Read the model definition and answer for the solid it produces. Units are mm, in the model's axes. A direction names the side the tool comes from. Round coordinates to 2 decimals unless told otherwise and drop trailing zeros. Write each loop counter-clockwise with the first axis right and the second up, starting at its lowest first coordinate (ties: lowest second). Pieces come first, ordered by that corner, then holes. Notation, with made-up numbers: (14.5, 22.5) -> (55.5, 22.5) arc R7 ccw to (55.5, 30.5) -> close; hole circle Ø5 at (-35, -32). An arc over 180 degrees is marked (long way). Return JSON: item names as keys, results as strings. Group by question number.
(1) Given pin 1 (1 mm diameter, centred on y = 4.5, z = 21.5, fed in from -X), flat-ended and moving along its own axis, determine where the tip first touches the part or whether it passes through.
(2) Straight lines are drawn through the part: line 1 (X direction, y = 0.25, z = 16.5); line 2 (Z direction, x = 4.25, y = 4.75); line 3 (Y direction, x = 0, z = -11.5). For each, find the intervals that lie inside material, in ascending order.
(3) The mould has two halves that part along Y. Classify faces 1 (the flat face through (0, 6.35, 1)), 2 (the cylindrical face through (1.926, 0.607, 1.451)), 3 (the flat face through (3, -6, 67.443)): released by +Y, released by -Y, zero draft, split by the parting line, or undercut.
(4) A cutting plane is placed at A-A on z = -51.5. Give the vertices of the cut face in (x, y) (3 decimals), then the cut area to 3 significant figures.
(5) For faces 4 (the flat face through (-1, 2, 67.443)), 5 (the flat face through (-3, 6, 67.443)), 6 (the flat face through (-3, -6, 67.443)), determine the directions among +Z, -Z, +X, -X, +Y, -Y from which every point of the face is accessible in a straight line to the end or side of a thin tool.
```python
from build123d import *

# Parameters (mm, degrees)
BOSS_EXTRUDE1_DEPTH              = 67.44335
SKETCH4_R                        = 6.35
SKETCH4_R_2                      = 2.4892
BOSS_EXTRUDE2_DEPTH              = 7.9375
F_10_32_TAPPED_HOLE1_D           = 4.0386
F_10_32_TAPPED_HOLE1_CSINK_D     = 6.096
F_10_32_TAPPED_HOLE1_CSINK_ANGLE = 90


with BuildPart() as part:
    # Sketch1 → Boss-Extrude1 (new, symmetric)
    with BuildSketch(Plane.XY):
        with BuildLine():
            ThreePointArc((4.181770846, 5.456960429), (3.437499983, 5.953924622), (2.634980936, 6.35))
            Line((2.634980936, 6.35), (-2.634980936, 6.35))
            ThreePointArc((-2.634980936, 6.35), (-3.437499983, 5.953924622), (-4.181770846, 5.456960429))
            Line((-4.181770846, 5.456960429), (-6.816751782, 0.893039571))
            ThreePointArc((-6.816751782, 0.893039571), (-6.874999966, 0), (-6.816751782, -0.893039571))
            Line((-6.816751782, -0.893039571), (-4.181770846, -5.456960429))
            ThreePointArc((-4.181770846, -5.456960429), (-3.437499983, -5.953924622), (-2.634980936, -6.35))
            Line((-2.634980936, -6.35), (2.634980936, -6.35))
            ThreePointArc((2.634980936, -6.35), (3.437499983, -5.953924622), (4.181770846, -5.456960429))
            Line((4.181770846, -5.456960429), (6.816751782, -0.893039571))
            ThreePointArc((6.816751782, -0.893039571), (6.860422465, -0.447468582), (6.874999966, 0))
            ThreePointArc((6.874999966, 0), (6.860422465, 0.447468582), (6.816751782, 0.893039571))
            Line((6.816751782, 0.893039571), (4.181770846, 5.456960429))
        make_face()
    extrude(amount=BOSS_EXTRUDE1_DEPTH, both=True)

    # Sketch4 → Boss-Extrude2 (add)
    with BuildSketch(Plane.XY.offset(67.44335)):
        with Locations(Location((0, 0, 0), (0, 0, 150))):
            Circle(SKETCH4_R)
        Circle(SKETCH4_R_2, mode=Mode.SUBTRACT)
    extrude(amount=BOSS_EXTRUDE2_DEPTH)

    # #10-32 Tapped Hole1 (through all)
    with Locations(Plane(origin=(0, 0, -67.44335), x_dir=(-1, 0, 0), z_dir=(0, 0, -1))):
        with Locations((0, 0)):
            CounterSinkHole(F_10_32_TAPPED_HOLE1_D / 2, F_10_32_TAPPED_HOLE1_CSINK_D / 2, counter_sink_angle=F_10_32_TAPPED_HOLE1_CSINK_ANGLE)


solid = part.part
```
Checks:
{
 "1": {"pin 1": "stops at x = -5.02"},
 "2": {"line 1": "x = -6.87 to -2, 2 to 6.87", "line 2": "z = -67.44 to 67.44", "line 3": "y = -6.35 to -2.02, 2.02 to 6.35"},
 "3": {"face 1": "released by +Y", "face 2": "undercut", "face 3": "zero draft"},
 "4": {"outline": "(-6.817, -0.893) -> (-4.182, -5.457) arc R6.875 ccw to (-2.635, -6.35) -> (2.635, -6.35) arc R6.875 ccw to (4.182, -5.457) -> (6.817, -0.893) arc R6.875 ccw to (6.817, 0.893) -> (4.182, 5.457) arc R6.875 ccw to (2.635, 6.35) -> (-2.635, 6.35) arc R6.875 ccw to (-4.182, 5.457) -> (-6.817, 0.893) arc R6.875 ccw to start; hole circle Ø4.039 at (0, 0)", "area": "125 mm^2"},
 "5": {"face 4": "+Z", "face 5": "+Z, -X, +Y", "face 6": "+Z, -X, -Y"}
}
